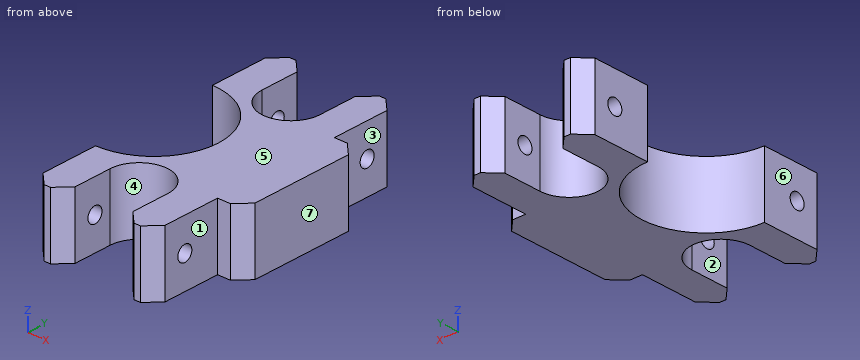
from build123d import *

# Parameters (mm, degrees)
BOSS_EXTRUDE1_DEPTH = 25
CUT_EXTRUDE1_DEPTH  = 50
SKETCH4_R           = 6
CUT_EXTRUDE2_DEPTH  = 200
CHAMFER1_SIZE       = 10
CHAMFER2_SIZE       = 10


with BuildPart() as part:
    # Sketch1 → Boss-Extrude1 (new, symmetric)
    with BuildSketch(Plane.XY):
        with BuildLine():
            Line((0, 50), (0, 105))
            Line((0, 105), (25, 105))
            Line((25, 105), (25, 65))
            Line((25, 65), (70, 65))
            Line((70, 65), (70, 105))
            Line((70, 105), (95, 105))
            Line((95, 105), (95, 50))
            Line((95, 50), (115, 50))
            Line((115, 50), (115, -50))
            Line((115, -50), (95, -50))
            Line((95, -50), (95, -105))
            Line((95, -105), (70, -105))
            Line((70, -105), (70, -65))
            Line((70, -65), (25, -65))
            Line((25, -65), (25, -105))
            Line((25, -105), (0, -105))
            Line((0, -105), (0, -50))
            ThreePointArc((0, -50), (50, 0), (0, 50))
        make_face()
    extrude(amount=BOSS_EXTRUDE1_DEPTH, both=True)

    # Sketch3 → Cut-Extrude1 (cut)
    with BuildSketch(Plane.XY.offset(25)):
        with BuildLine():
            Line((25, 65), (70, 65))
            ThreePointArc((70, 65), (47.5, 42.5), (25, 65))
        make_face()
        with BuildLine():
            Line((25, -65), (70, -65))
            ThreePointArc((70, -65), (47.5, -42.5), (25, -65))
        make_face()
    extrude(amount=-CUT_EXTRUDE1_DEPTH, mode=Mode.SUBTRACT)

    # Sketch4 → Cut-Extrude2 (cut)
    with BuildSketch(Plane.ZY):
        with Locations((0, 78)):
            Circle(SKETCH4_R)
        with Locations(Location((0, -78, 0), (0, 0, 270))):
            Circle(SKETCH4_R)
    extrude(amount=-CUT_EXTRUDE2_DEPTH, mode=Mode.SUBTRACT)

    # Chamfer1
    chamfer1_edges = [part.edges().sort_by_distance(p)[0] for p in [
        (115, 50, 0),
        (115, -50, 0),
    ]]
    chamfer(chamfer1_edges, length=CHAMFER1_SIZE)

    # Chamfer2
    chamfer2_edges = [part.edges().sort_by_distance(p)[0] for p in [
        (0, 105, 0),
        (25, 105, 0),
        (70, 105, 0),
        (95, 105, 0),
        (95, -105, 0),
        (70, -105, 0),
        (25, -105, 0),
        (0, -105, 0),
    ]]
    chamfer(chamfer2_edges, length=CHAMFER2_SIZE)


solid = part.part
Verification items for the finished model (mm, model axes). Face numbers are marked on the shaded views. A direction names the side the tool comes from. Round coordinates to 2 decimals unless told otherwise and drop trailing zeros. Loops run counter-clockwise (first coordinate to the right, second up) from the corner with the lowest first, then second, coordinate; pieces in that order, holes last. Notation, with made-up numbers: (-30.75, 7) - (9.25, 7) arc R15 ccw to (9.25, 12) - close; hole circle Ø6 at (66.5, 70). An arc over 180 degrees is marked (long way). Write item = value, one per line.
Q1. Sectioned sample at A-A on y = -68. Record the boundary of the cut face in (x, z), plus the area to 3 significant figures.
Here are the results:
outline = (0, -25) - (25, -25) - (25, 25) - (0, 25) - close; (70, -25) - (95, -25) - (95, 25) - (70, 25) - close
area = 2,500 mm^2
Q2. Sectioned sample at B-B on x = 72. Record the boundary of the cut face in (y, z).
Here are the results:
outline = (-97, -25) - (97, -25) - (97, 25) - (-97, 25) - close; hole circle Ø12 at (-78, 0); hole circle Ø12 at (78, 0)
Q3. Sectioned sample at C-C on z = -8. Record the boundary of the cut face in (x, y), plus the area to 3 significant figures.
Here are the results:
outline = (0, -95) - (10, -105) - (15, -105) - (25, -95) - (25, -65) arc R22.5 cw to (70, -65) - (70, -95) - (80, -105) - (85, -105) - (95, -95) - (95, -50) - (105, -50) - (115, -40) - (115, 40) - (105, 50) - (95, 50) - (95, 95) - (85, 105) - (80, 105) - (70, 95) - (70, 65) arc R22.5 cw to (25, 65) - (25, 95) - (15, 105) - (10, 105) - (0, 95) - (0, 50) arc R50 cw to (0, -50) - close
area = 12,300 mm^2
Q4. Depth check by flat-ended pin: pin 1 (13.5 mm diameter, centred on y = 68.5, z = 9.5, fed in from +X); pin 2 (11 mm diameter, centred on y = -78, z = 0, fed in from +X); pin 3 (8 mm diameter, centred on x = 31, z = -4.5, fed in from +Y); pin 4 (2 mm diameter, centred on x = 24, z = -6.5, fed in from +Y). Enter the tip coordinate at first touch or a pass-through.
Here are the results:
pin_1 = 95
pin_2 = through
pin_3 = 55.73
pin_4 = 97
Q5. Sectioned sample at D-D on x = 19. Record the boundary of the cut face in (y, z).
Here are the results:
outline = (-101, -25) - (-46.25, -25) - (-46.25, 25) - (-101, 25) - close; (46.25, -25) - (101, -25) - (101, 25) - (46.25, 25) - close; hole circle Ø12 at (-78, 0); hole circle Ø12 at (78, 0)
Q6. Tool access check on the marked faces 1, 2 and 3. Record the directions out of +Z, -Z, +X, -X, +Y, -Y that give a thin tool (end or side, any length) a straight path to the whole face; none if there is none.
Here are the results:
face_1 = +Z, -Z, +X, -Y
face_2 = +Z, -Z, -Y
face_3 = +Z, -Z, +X, +Y
Q7. Material ranges on L1, parallel to X at y = -88.5, z = -18.5; L2, parallel to Y at x = 22, z = 4; L3, parallel to Y at x = 102.5, z = -21, recorded low to high.
Here are the results:
L1 = 0 to 25, 70 to 95
L2 = -98 to -82.47, -73.53 to -44.9, 44.9 to 73.53, 82.47 to 98
L3 = -50 to 50
Q8. Mould release check, pull along X, two halves, no side actions. Record for the marked faces 4, 5, 6 and 7: +X half, -X half, draft (parallel to the pull), parting line (faces both ways), or undercut.
Here are the results:
face_4 = undercut
face_5 = draft
face_6 = -X half
face_7 = +X half
